from build123d import *

# Parameters (mm, degrees)
SKETCH_1_W          = 12
SKETCH_1_H          = 12
EXTRUDE_1_DEPTH     = 40
SKETCH_2_W          = 10
SKETCH_2_H          = 10
CUT_EXTRUDE_1_DEPTH = 47.5
SKETCH_3_R          = 2.1
CUT_EXTRUDE_2_DEPTH = 47.5
SKETCH_5_R          = 3.5
CUT_EXTRUDE_4_DEPTH = 47.5


with BuildPart() as part:
    # ｽｹｯﾁ1 → ﾎﾞｽ - 押し出し1 (new body)
    with BuildSketch(Plane.XY):
        Rectangle(SKETCH_1_W, SKETCH_1_H)
    extrude(amount=EXTRUDE_1_DEPTH)

    # ｽｹｯﾁ2 → ｶｯﾄ - 押し出し1 (cut)
    with BuildSketch(Plane.XY.offset(40)):
        Rectangle(SKETCH_2_W, SKETCH_2_H)
    extrude(amount=-CUT_EXTRUDE_1_DEPTH, mode=Mode.SUBTRACT)

    # ｽｹｯﾁ3 → ｶｯﾄ - 押し出し2 (cut)
    with BuildSketch(Plane(origin=(0, 6, 0), x_dir=(1, 0, 0), z_dir=(0, 1, 0))):
        with Locations((0, -5)):
            Circle(SKETCH_3_R)
        with Locations((0, -35)):
            Circle(SKETCH_3_R)
    extrude(amount=-CUT_EXTRUDE_2_DEPTH, mode=Mode.SUBTRACT)

    # ｽｹｯﾁ5 → ｶｯﾄ - 押し出し4 (cut)
    with BuildSketch(Plane.ZY.offset(6)):
        with Locations((35, 0)):
            Circle(SKETCH_5_R)
    extrude(amount=-CUT_EXTRUDE_4_DEPTH, mode=Mode.SUBTRACT)


solid = part.part
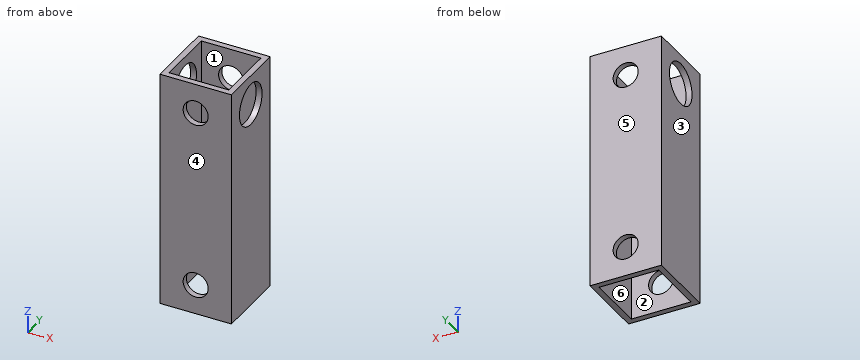
Check sheet for the modelled part. Datum: model origin and axes. Units: mm. Face numbers are marked on the shaded views. A direction names the side the tool comes from. Round coordinates to 2 decimals unless told otherwise and drop trailing zeros. Loops run counter-clockwise (first coordinate to the right, second up) from the corner with the lowest first, then second, coordinate; pieces in that order, holes last. Notation, with made-up numbers: M 8,64 L 38,64 A31 cw 38,89 Z; hole C 42,-14 d2. An arc over 180 degrees is marked long. One line per question, with ' | ' between items. Start each with the question number.
Item 1: Section check D-D (y = 0). Record the boundary of the cut face in (x, z).
Item 2: Scan lines: probe 1 along Z at (x, y) = (0, 5.5); probe 2 along Y at (x, z) = (0.75, 10.5). Record each from-to range of solid material in increasing order.
Item 3: Section check C-C (x = 3.5). Record the boundary of the cut face in (y, z), and give its area (3 significant figures).
Item 4: Section check B-B (z = 35). Record the boundary of the cut face in (x, y).
Item 5: Set-up check for the marked faces 5 and 6: record each of +Z, -Z, +X, -X, +Y, -Y from which the full face is reachable in a straight line by a thin tool's end or side.
Item 6: Release check for a two-part mould opening along Y. For the marked faces 1, 2, 3 and 4 record: released by +Y, released by -Y, zero draft, split by the parting line, or undercut.
Item 7: Section check A-A (x = 0). Record the boundary of the cut face in (y, z).
Worked out:
1) outline: M -6,0 L -5,0 L -5,31.5 L -6,31.5 Z; M -6,38.5 L -5,38.5 L -5,40 L -6,40 Z; M 5,0 L 6,0 L 6,31.5 L 5,31.5 Z; M 5,38.5 L 6,38.5 L 6,40 L 5,40 Z
2) probe 1: 0 to 2.9, 7.1 to 32.9, 37.1 to 40 | probe 2: -6 to -5, 5 to 6
3) outline: M -6,0 L -5,0 L -5,40 L -6,40 Z; M 5,0 L 6,0 L 6,40 L 5,40 Z | area: 80.0 mm^2
4) outline: M -6,-6 L -2.1,-6 L -2.1,-5 L -5,-5 L -5,-3.5 L -6,-3.5 Z; M -6,3.5 L -5,3.5 L -5,5 L -2.1,5 L -2.1,6 L -6,6 Z; M 2.1,-6 L 6,-6 L 6,-3.5 L 5,-3.5 L 5,-5 L 2.1,-5 Z; M 2.1,5 L 5,5 L 5,3.5 L 6,3.5 L 6,6 L 2.1,6 Z
5) face 5: +Z, -Z, +X, -X, +Y | face 6: +Z, -Z
6) face 1: undercut | face 2: undercut | face 3: zero draft | face 4: released by -Y
7) outline: M -6,0 L -5,0 L -5,2.9 L -6,2.9 Z; M -6,7.1 L -5,7.1 L -5,32.9 L -6,32.9 Z; M -6,37.1 L -5,37.1 L -5,40 L -6,40 Z; M 5,0 L 6,0 L 6,2.9 L 5,2.9 Z; M 5,7.1 L 6,7.1 L 6,32.9 L 5,32.9 Z; M 5,37.1 L 6,37.1 L 6,40 L 5,40 Z
